Here's the drawing with two shaded views (mm, measured from the low corner). I have some questions. Round coordinates to 2 decimals unless told otherwise and drop trailing zeros. Write each loop counter-clockwise with the first axis right and the second up, starting at its lowest first coordinate (ties: lowest second). Pieces come first, ordered by that corner, then holes. Notation, with made-up numbers: M 27,78 L 64,78 A21 ccw 64,114 Z; hole C 23.5,79 d6. An arc over 180 degrees is marked long. Answer as a JSON object with one key per item and string values. Group by question number.
1) Suppose I cut it at B-B, the plane z = 27.5. Write out the boundary of the cut face in (x, y), and give its area (3 significant figures).
2) Suppose I cut it at A-A, the plane z = 42. Write out the boundary of the cut face in (x, y).
3) I'm going to push flat-ended pins straight in: pin 1 Ø2 at (x, z) = (11.96, 15.68) entering from +Y; pin 2 Ø1.4 at (y, z) = (1.5, 41.5) entering from -X. Where does each tip first touch, or does it pass through?
4) Suppose I cut it at C-C, the plane y = 1.7. State how many separate pieces and enclosed holes the cut face has, and give its area (3 significant figures).
5) Please list where these lines run through material, in increasing order: L1, parallel to X at y = 2.45, z = 32; L2, parallel to Z at x = 20, y = 2.35; L3, parallel to Z at x = 10, y = 2.4 (1 decimal). Write a range as [from, to].
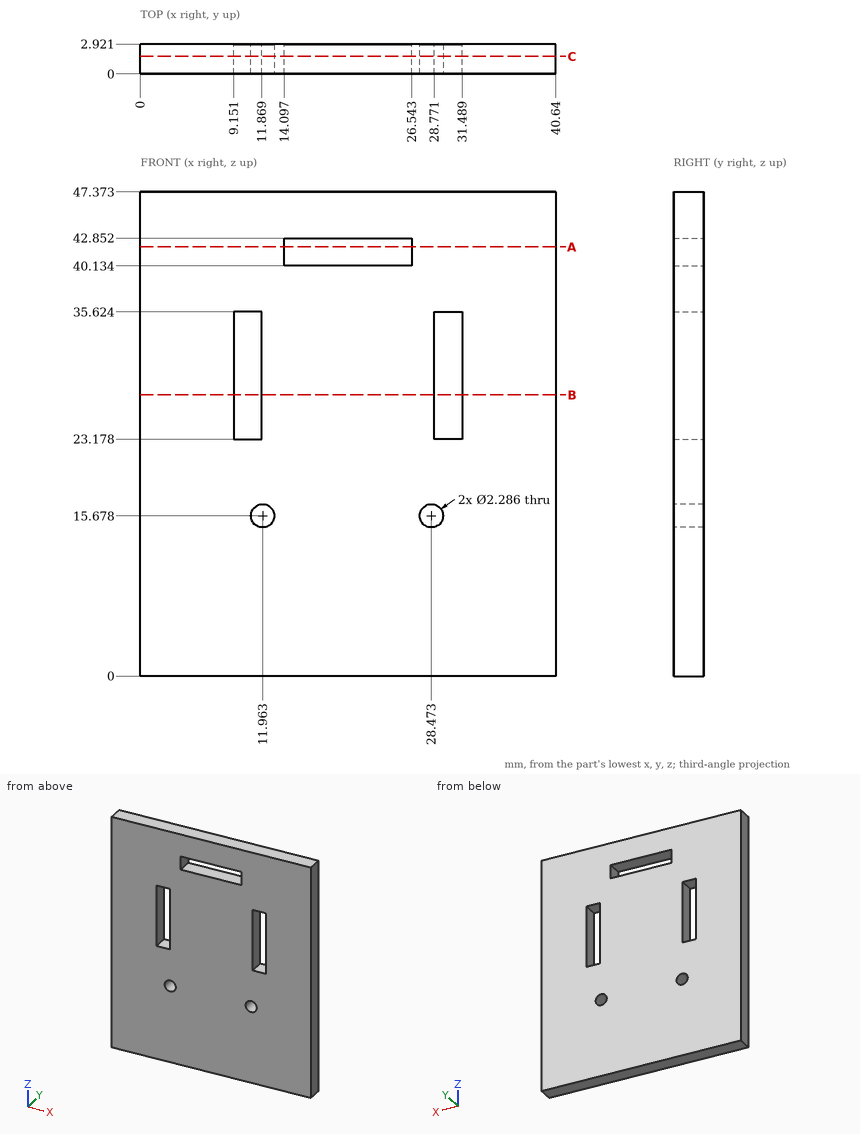
Results:
{
 "1": {"outline": "M 0,0 L 9.15,0 L 9.15,2.92 L 0,2.92 Z; M 11.87,0 L 28.77,0 L 28.77,2.92 L 11.87,2.92 Z; M 31.49,0 L 40.64,0 L 40.64,2.92 L 31.49,2.92 Z", "area": "103 mm^2"},
 "2": {"outline": "M 0,0 L 14.1,0 L 14.1,2.92 L 0,2.92 Z; M 26.54,0 L 40.64,0 L 40.64,2.92 L 26.54,2.92 Z"},
 "3": {"pin 1": "through", "pin 2": "x = 0"},
 "4": {"separate pieces": "1", "enclosed holes": "5", "area": "1,820 mm^2"},
 "5": {"L1": "[0, 9.15], [11.87, 28.77], [31.49, 40.64]", "L2": "[0, 40.13], [42.85, 47.37]", "L3": "[0, 23.2], [35.6, 47.4]"}
}
